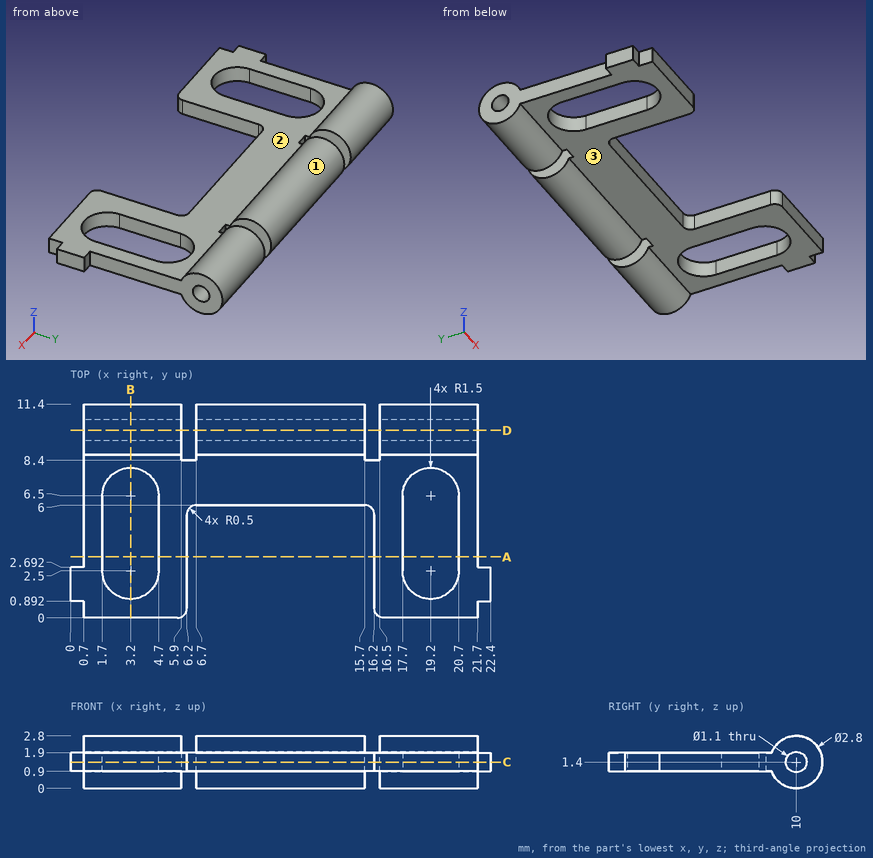
Part print with two shaded views. Sizes in mm from the minimum x, y, z corner. A direction names the side the tool comes from. Give positions to 0.01 mm unless a question says otherwise; leave off trailing zeros. Loops run counter-clockwise (first coordinate to the right, second up) from the corner with the lowest first, then second, coordinate; pieces in that order, holes last. Notation, with made-up numbers: (46.25, 3.5) - (86.25, 3.5) arc R19 cw to (86.25, 37.5) - close; hole circle Ø10 at (78.5, 81.25). An arc over 180 degrees is marked (long way). Put each result on its own line as item: value.
Q1. Slice it at A-A (y = 3.25). Give the cut face in (x, z).
Filled in:
outline: (0.7, 0.9) - (1.7, 0.9) - (1.7, 1.9) - (0.7, 1.9) - close; (4.7, 0.9) - (6.2, 0.9) - (6.2, 1.9) - (4.7, 1.9) - close; (16.2, 0.9) - (17.7, 0.9) - (17.7, 1.9) - (16.2, 1.9) - close; (20.7, 0.9) - (21.7, 0.9) - (21.7, 1.9) - (20.7, 1.9) - close
Q2. Flat gauge pins, fed straight in: pin 1 (1.5 mm diameter, centred on x = 6, z = 0.5, fed in from +Y); pin 2 (1.1 mm diameter, centred on x = 11.5, z = 1, fed in from -Y); pin 3 (1.4 mm diameter, centred on y = 10.5, z = 2, fed in from -X); pin 4 (1 mm diameter, centred on x = 11.5, y = 5, fed in from +Z). Where does each tip first touch, or does it go through?
Filled in:
pin 1: stops at y = 11.39
pin 2: stops at y = 6
pin 3: stops at x = 0.7
pin 4: passes through
Q3. Probe line 1 along X through (y, z) = (10.5, 0.8); line 2 along X through (y, z) = (5.25, 1.65); line 3 along Z through (x, y) = (19.95, 10). List the from-to ranges inside material, lowest first.
Filled in:
line 1: x = 0.7 to 5.9, 6.7 to 15.7, 16.5 to 21.7
line 2: x = 0.7 to 1.7, 4.7 to 6.2, 16.2 to 17.7, 20.7 to 21.7
line 3: z = 0 to 0.85, 1.95 to 2.8
Q4. Slice it at C-C (z = 1.4). Give the number of separate pieces and of enclosed holes in the cut face, plus the area to 3 significant figures.
Filled in:
separate pieces: 4
enclosed holes: 2
area: 118 mm²
Q5. Tool access for the marked faces 1, 2 and 3: list every direction of +Z, -Z, +X, -X, +Y, -Y with a clear straight run to the whole face (end or side of a thin tool).
Filled in:
face 1: +X, -X
face 2: +Z, +X, -X, -Y
face 3: -Z, +X, -X, -Y
Q6. Slice it at B-B (x = 3.2). Give the cut face in (y, z).
Filled in:
outline: (0, 0.9) - (1, 0.9) - (1, 1.9) - (0, 1.9) - close; (8, 0.9) - (8.69, 0.9) arc R1.4 ccw (long way) to (8.69, 1.9) - (8, 1.9) - close; hole circle Ø1.1 at (10, 1.4)
Q7. Slice it at D-D (y = 10). Give the cut face in (x, z).
Filled in:
outline: (0.7, 0) - (5.9, 0) - (5.9, 0.85) - (0.7, 0.85) - close; (0.7, 1.95) - (5.9, 1.95) - (5.9, 2.8) - (0.7, 2.8) - close; (6.7, 0) - (15.7, 0) - (15.7, 0.85) - (6.7, 0.85) - close; (6.7, 1.95) - (15.7, 1.95) - (15.7, 2.8) - (6.7, 2.8) - close; (16.5, 0) - (21.7, 0) - (21.7, 0.85) - (16.5, 0.85) - close; (16.5, 1.95) - (21.7, 1.95) - (21.7, 2.8) - (16.5, 2.8) - close
